Geometry: see drawing. Coordinates: mm, zero at the bounding-box minimum. Give positions to 0.01 mm unless a question says otherwise; leave off trailing zeros. Order: outer loops, then holes, each group sorted by start corner. A loop starts at its lowest first (then second) coordinate and runs counter-clockwise, first axis right, second up. Notation, with made-up numbers: (82, -12) - (123, -12) arc R19 ccw to (123, 8) - close; hole circle Ø5 at (3, -29). An arc over 180 degrees is marked (long way). Put each result on its own line as item: value. Start each with the question number.
1. Section A-A on z = 11.25. Return the cut outline in (x, y), plus the area to 3 significant figures.
2. Mould query, pull axis Z, two halves, no side actions, for the marked faces 1, 2 and 3. Classes: pulls with the +Z half, pulls with the -Z half, needs draft (parallel to the pull), parting line crosses it, or undercut.
3. Section B-B on x = 11.25. Return the cut outline in (y, z).
4. Section C-C on y = 2.5. Return the cut outline in (x, z).
5. Ray query, line 1 along X through (y, z) = (1.75, 11.25); line 2 along X through (y, z) = (5.7, 11.25); line 3 along Y through (x, z) = (15.75, 19). Return the intervals inside material, ascending. Write a range as from..to.
6. First-contact query: P1, Ø3, axis at y = 2, z = 2.5, coming from the +X side; P2, Ø10, axis at x = 8, z = 7.5, coming from the +Y side; P3, Ø13, axis at x = 11.25, z = 11.25, coming from the +Y side. Flat tips, straight axial feed; report the tip coordinate or a pass-through.
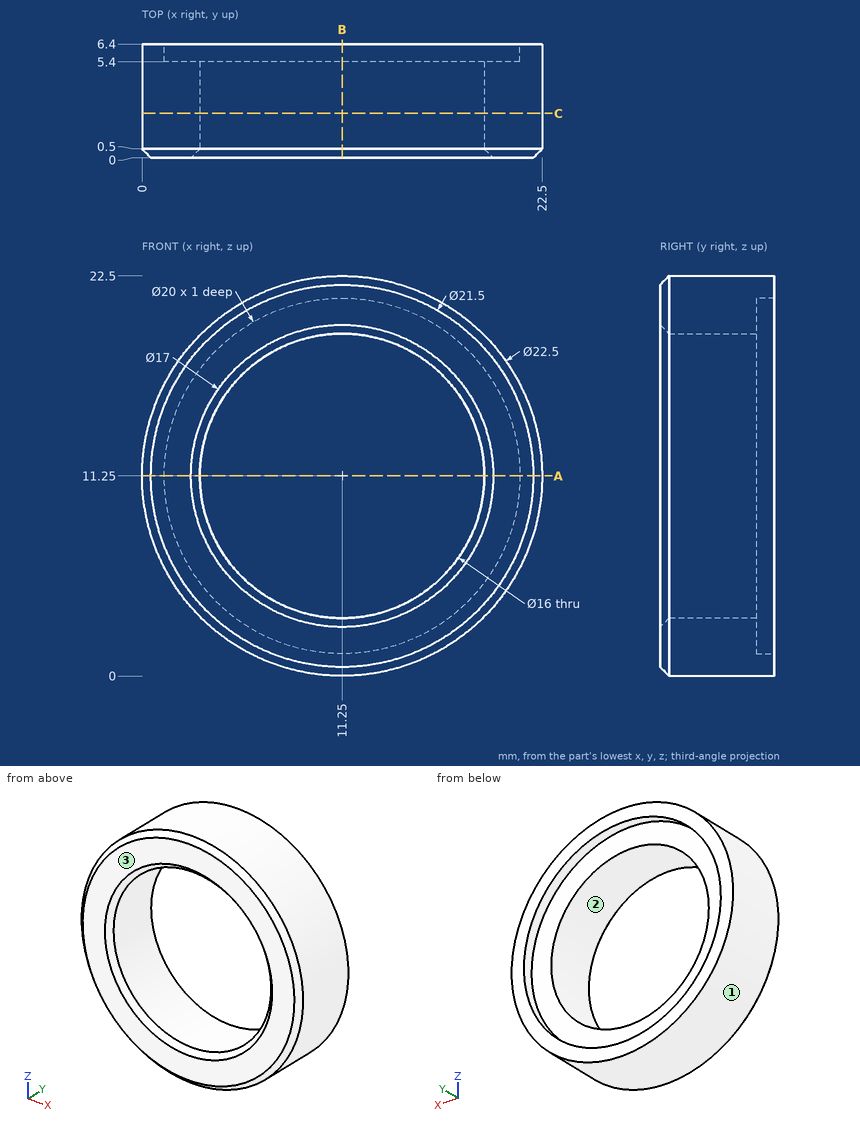
Resolved:
1. outline: (0, 0.5) - (0.5, 0) - (2.75, 0) - (3.25, 0.5) - (3.25, 5.4) - (1.25, 5.4) - (1.25, 6.4) - (0, 6.4) - close; (19.25, 0.5) - (19.75, 0) - (22, 0) - (22.5, 0.5) - (22.5, 6.4) - (21.25, 6.4) - (21.25, 5.4) - (19.25, 5.4) - close
1. area: 37.1 mm^2
2. face 1: parting line crosses it
2. face 2: undercut
2. face 3: needs draft
3. outline: (0, 0.5) - (0.5, 0) - (6.4, 0) - (6.4, 1.25) - (5.4, 1.25) - (5.4, 3.25) - (0.5, 3.25) - (0, 2.75) - close; (0, 19.75) - (0.5, 19.25) - (5.4, 19.25) - (5.4, 21.25) - (6.4, 21.25) - (6.4, 22.5) - (0.5, 22.5) - (0, 22) - close
4. outline: circle Ø22.5 at (11.25, 11.25); hole circle Ø16 at (11.25, 11.25)
5. line 1: 0..3.25, 19.25..22.5
5. line 2: 0..1.25, 21.25..22.5
5. line 3: 0..5.4
6. P1: x = 19.85
6. P2: y = 5.4
6. P3: through
